Part print with two shaded views. Sizes in mm from the minimum x, y, z corner. Give positions to 0.01 mm unless a question says otherwise; leave off trailing zeros. Order: outer loops, then holes, each group sorted by start corner. A loop starts at its lowest first (then second) coordinate and runs counter-clockwise, first axis right, second up.
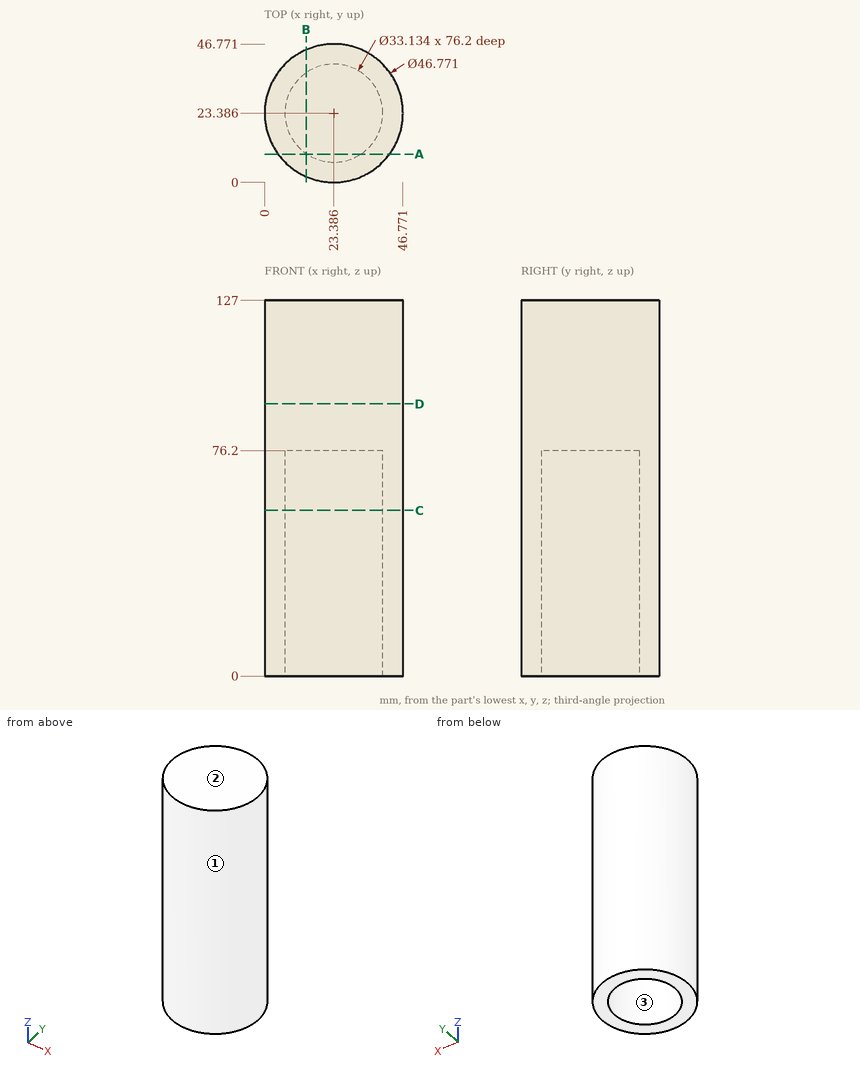
Item 1: Wall check: L1, parallel to Z at x = 14, y = 20.5; L2, parallel to X at y = 11.5, z = 41 (1 decimal); L3, parallel to Y at x = 19, z = 61 (1 decimal). Give the ranges that are in metal, low to high.
Item 2: Slice it at D-D (z = 92). Give the cut face in (x, y) (1 decimal).
Item 3: Drop flat-ended pins along their axis: pin 1 Ø6 at (x, y) = (11.5, 18) entering from -Z; pin 2 Ø10 at (x, z) = (33, 36.5) entering from -Y; pin 3 Ø4 at (x, z) = (28.5, 58.5) entering from +Y; pin 4 Ø5 at (x, y) = (42, 30.5) entering from -Z. Give the stop position or say it passes through.
Item 4: Two-plate mould, pull along Y, no slides. Class the marked faces 1, 2 and 3: released by +Y, released by -Y, zero draft, split by the parting line, or undercut.
Item 5: Slice it at B-B (x = 14). Give the cut face in (y, z) (1 decimal).
Item 6: Slice it at C-C (z = 56). Give the cut face in (x, y) (1 decimal).
Item 7: Slice it at A-A (y = 9.5). Give the cut face in (x, z), and give its area (3 significant figures).
A:
1. L1: z = 76.2 to 127
1. L2: x = 3.2 to 11.8, 34.9 to 43.5
1. L3: y = 0.4 to 7.4, 39.4 to 46.4
2. outline: circle Ø46.8 at (23.4, 23.4)
3. pin 1: stops at z = 76.2
3. pin 2: stops at y = 0.46
3. pin 3: stops at y = 46.56
3. pin 4: stops at z = 0
4. face 1: split by the parting line
4. face 2: zero draft
4. face 3: undercut
5. outline: (2, 0) - (9.7, 0) - (9.7, 76.2) - (37, 76.2) - (37, 0) - (44.8, 0) - (44.8, 127) - (2, 127) - close
6. outline: circle Ø46.8 at (23.4, 23.4); hole circle Ø33.1 at (23.4, 23.4)
7. outline: (4.57, 0) - (14.35, 0) - (14.35, 76.2) - (32.42, 76.2) - (32.42, 0) - (42.2, 0) - (42.2, 127) - (4.57, 127) - close
7. area: 3,400 mm2
